Work out the finished part from the listing and answer in its coordinate system (mm). A direction names the side the tool comes from. Coordinates: 2 decimals unless noted, no trailing zeros. Order: outer loops, then holes, each group sorted by start corner. A loop starts at its lowest first (then second) coordinate and runs counter-clockwise, first axis right, second up. Notation, with made-up numbers: (89, 84) -> (114, 84) arc R24 ccw to (114, 115) -> close; hole circle Ø9 at (-23, 55.5). An arc over 180 degrees is marked (long way). Use one line per item in the form item = value.
Autodesk Inventor part; units mm, degrees
ref_plane "YZ Plane" through (0, 0, 0) normal (1, 0, 0) x (0, 1, 0)
ref_plane "XZ Plane" through (0, 0, 0) normal (0, 1, 0) x (-1, 0, 0)
ref_plane "XY Plane" through (0, 0, 0) normal (0, 0, 1) x (1, 0, 0)
sketch "Sketch1" plane through (0, 0, 0) normal (0, 1, 0) x (-1, 0, 0)
  line L0 (0, 0) -> (12.71, 0) construction
  line L1 (12.71, 25.41) -> (-12.71, 25.41)
  line L2 (-12.71, 25.41) -> (-12.71, -25.41)
  line L3 (-12.71, -25.41) -> (12.71, -25.41)
  line L4 (12.71, 25.41) -> (12.71, -25.41)
  dimension "d0" = 12.71
  dimension "d1" = 25.41
  dimension "d2" = 25.42
  dimension "d3" = 50.82
extrude "Extrusion1" add sketch "Sketch1" along normal mid plane 12.6
sketch "Sketch2" plane through (0, -6.3, 0) normal (0, -1, 0) x (1, 0, 0)
  line L0 (12.71, 25.41) -> (12.71, 20.31) construction
  line L1 (12.71, 20.31) -> (6.26, 20.31)
  line L2 (12.71, -25.41) -> (12.71, -20.31) construction
  line L3 (12.71, -20.31) -> (6.26, -20.31)
  line L4 (6.26, -20.31) -> (6.26, 20.31)
  line L5 (12.71, 20.31) -> (12.71, -20.31)
  line L6 (12.71, 25.41) -> (12.71, -25.41)
  line L7 (0, 25.41) -> (0, -25.41)
  line L8 (-12.71, 20.31) -> (-6.26, 20.31)
  line L9 (-12.71, -20.31) -> (-6.26, -20.31)
  line L10 (-6.26, -20.31) -> (-6.26, 20.31)
  line L11 (-12.71, 20.31) -> (-12.71, -20.31)
  point P0 (0, 0)
  dimension "d6" = 5.1
  dimension "d7" = 6.45
  dimension "d8" = 5.1
  dimension "d9" = 6.45
extrude "Extrusion2" cut sketch "Sketch2" against normal blind 6.25
fillet "Fillet1" radius 4 4 edges at (6.26, -3.175, 20.31) (6.26, -3.175, -20.31) (-6.26, -3.175, -20.31) (-6.26, -3.175, 20.31)
sketch "Sketch3" plane through (0, 6.3, 0) normal (0, 1, 0) x (1, 0, 0)
  line L0 (-12.71, 25.41) -> (-12.71, 22.91) construction
  line L1 (-12.71, 22.91) -> (-10.21, 22.91) construction
  circle A0 centre (-10.21, 22.91) radius 1.5
  circle A1 centre (-10.21, -17.09) radius 1.5
  circle A2 centre (-10.21, -12.09) radius 1.5
  circle A3 centre (-10.21, -7.09) radius 1.5
  circle A4 centre (-10.21, -2.09) radius 1.5
  circle A5 centre (-10.21, 2.91) radius 1.5
  circle A6 centre (-10.21, 7.91) radius 1.5
  circle A7 centre (-10.21, 12.91) radius 1.5
  circle A8 centre (-10.21, 17.91) radius 1.5
  circle A9 centre (10.21, 22.91) radius 1.5
  circle A10 centre (10.21, -17.09) radius 1.5
  circle A11 centre (10.21, -12.09) radius 1.5
  circle A12 centre (10.21, -7.09) radius 1.5
  circle A13 centre (10.21, -2.09) radius 1.5
  circle A14 centre (10.21, 2.91) radius 1.5
  circle A15 centre (10.21, 7.91) radius 1.5
  circle A16 centre (10.21, 12.91) radius 1.5
  circle A17 centre (10.21, 17.91) radius 1.5
  circle A18 centre (0, 21.91) radius 1.75 construction
  line L2 (0, 0) -> (0, 21.91) construction
  line L3 (0, 0) -> (0, -21.91) construction
  circle A19 centre (0, -21.91) radius 1.75 construction
  circle A20 centre (0, -21.91) radius 1.5
  circle A21 centre (0, 21.91) radius 1.5
  line L4 (0, -21.91) -> (0, 1.95) construction
  circle A22 centre (0, 1.95) radius 2.2
  dimension "d13" = 2.5
  dimension "d15" = 3
  dimension "d25" = 3
  dimension "d26" = 3
  dimension "d27" = 3
  dimension "d28" = 3
  dimension "d29" = 3
  dimension "d30" = 3
  dimension "d31" = 3
  dimension "d32" = 3
  dimension "d33" = 5
  dimension "d35" = 3.5
  dimension "d36" = 21.91
  dimension "d38" = 21.91
  dimension "d39" = 3.5
  dimension "d40" = 3
  dimension "d41" = 3
  dimension "d42" = 23.86
  dimension "d43" = 4.4
extrude "Extrusion3" cut sketch "Sketch3" against normal blind 15.775
sketch "Sketch4" plane through (0, 6.3, 0) normal (0, 1, 0) x (1, 0, 0)
  circle A0 centre (0, -21.91) radius 1.75
  circle A1 centre (0, 21.91) radius 1.75
  point P0 (0, 0)
  dimension "d46" = 3.5
  dimension "d47" = 3.5
extrude "Extrusion4" cut sketch "Sketch4" against normal blind 4.6
sketch "Sketch5" plane through (0, 6.3, 0) normal (0, 1, 0) x (1, 0, 0)
  circle A0 centre (0, 1.95) radius 3.65
  point P0 (0, 0)
  dimension "d50" = 7.3
extrude "Extrusion5" cut sketch "Sketch5" against normal blind 5.7
sketch "Sketch6" plane through (-12.71, 6.3, 25.41) normal (0, 0, 1) x (1, 0, 0)
  line L0 (25.42, -12.6) -> (22.07, -12.6) construction
  line L1 (22.07, -12.6) -> (22.07, -9.25) construction
  circle A0 centre (22.07, -9.25) radius 2.35
  line L2 (12.71, -0.1064) -> (12.71, -12.6)
  circle A1 centre (3.35, -9.25) radius 2.35
  circle A2 centre (12.71, -6.3) radius 2.425
  dimension "d53" = 3.35
  dimension "d54" = 3.35
  dimension "d55" = 4.7
  dimension "d56" = 4.85
extrude "Extrusion6" cut sketch "Sketch6" against normal blind 13.5
properties part number "PocketNC_Vise_part2" material "Aluminum 6061"
(1) Each of these flat-tipped pins is pushed along its axis until it touches: P1, Ø4, axis at x = 10.21, z = 7.09, coming from the -Y side; P2, Ø4, axis at x = -9.36, y = -2.95, coming from the +Z side (3 decimals); P3, Ø3, axis at y = -5, z = 2.5, coming from the -X side. Where does it stop, or does it pass through?
Data:
P1 = -0.05
P2 = -19.065
P3 = -6.26
(2) Section A-A on z = -12.91 is taken. Write down the section's boundary in (x, y), plus the area to 3 significant figures.
Data:
outline = (-12.71, -0.05) -> (-11.71, -0.05) -> (-11.71, 6.3) -> (-12.71, 6.3) -> close; (-8.71, -0.05) -> (-6.26, -0.05) -> (-6.26, -6.3) -> (6.26, -6.3) -> (6.26, -0.05) -> (8.71, -0.05) -> (8.71, 6.3) -> (-8.71, 6.3) -> close; (11.71, -0.05) -> (12.71, -0.05) -> (12.71, 6.3) -> (11.71, 6.3) -> close
area = 202 mm²
(3) Section B-B on x = 0 is taken. Count the separate pieces of the cut face and the enclosed holes in it, plus the area to 3 significant figures.
Data:
separate_pieces = 5
enclosed_holes = 0
area = 438 mm²
(4) Section D-D on z = 15 is taken. Write down the section's boundary in (x, y) (3 decimals).
Data:
outline = (-12.71, -0.05) -> (-6.26, -0.05) -> (-6.26, -6.3) -> (6.26, -6.3) -> (6.26, -0.05) -> (12.71, -0.05) -> (12.71, 6.3) -> (-12.71, 6.3) -> close; hole circle Ø4.85 at (0, 0)
(5) Which of the six approach directions +Z, -Z, +X, -X, +Y, -Y give full straight-line access (tool end or side, diameter ignored) to faces 1 (the cylindrical face through (-0.38, 4.03, -20.2)), 2 (the cylindrical face through (7.463, -3.131, -19.169)), 3 (the cylindrical face through (-7.12, -2.24, 22.83)), 4 (the flat face through (0, 0, -25.41)), 5 (the cylindrical face through (10.9, 0.09, -21.58))?
Data:
face_1 = +Y
face_2 = +X, -Y
face_3 = +Z
face_4 = -Z, +X, -X, +Y, -Y
face_5 = +Y, -Y
(6) Straight lines are drawn through the part: line 1 along X through (y, z) = (1.75, -12.91); line 2 along X through (y, z) = (-2.95, 22); line 3 along X through (y, z) = (4.6, 21.91). For each, find the intervals that lie inside material, in ascending order.
Data:
line_1 = -12.71 to -11.71, -8.71 to 8.71, 11.71 to 12.71
line_2 = -12.71 to -11.71, -7.01 to -1.5, 1.5 to 7.01, 11.71 to 12.71
line_3 = -12.71 to -1.75, 1.75 to 12.71
(7) The mould has two halves that part along Z. Classify faces 6 (the cylindrical face through (-7.401, -3.131, -19.107)), 7 (the flat face through (0, 3, 25.41)), 8 (the cylindrical face through (7.012, -2.847, 22.825)), 9 (the flat face through (12, -3, -20.31)): released by +Z, released by -Z, zero draft, split by the parting line, or undercut.
Data:
face_6 = undercut
face_7 = released by +Z
face_8 = zero draft
face_9 = undercut
